```python
from build123d import *

# Parameters (mm, degrees)
F4_DEPTH = 25.4


with BuildPart() as f1:
    # F0 (on Front) → F1 (revolve)
    with BuildSketch(Plane.XZ):
        Polygon((-83.82, 18.745402), (-83.82, 14.483047), (-88.9, 14.483047), (-88.9, 34.294205), (-107.182943, 34.294205), (-177.8, -87.390703), (-177.8, -95.645703), (-162.954339, -95.645703), (-133.013525, -44.052713), (-80.645, 4.534993), (-80.645, 18.745402), align=None)
    revolve(axis=Axis((0, 0, -6.240661), (0, 0, -1)))

    # F3 (on offset) → F4 (cut)
    with BuildSketch(Plane.XY.offset(8.894205)):
        Polygon((6.35, -86.36), (6.35, -66.04), (-6.35, -66.04), (-6.35, -86.36), (-6.35, -92.71), (6.35, -92.71), align=None)
        Polygon((-54.017318, 38.519261), (-71.614954, 48.679261), (-77.114215, 51.854261), (-83.464215, 40.855739), (-77.964954, 37.680739), (-60.367318, 27.520739), align=None)
        Polygon((60.367318, 27.520739), (77.964954, 37.680739), (83.464215, 40.855739), (77.114215, 51.854261), (71.614954, 48.679261), (54.017318, 38.519261), align=None)
    extrude(amount=-F4_DEPTH, mode=Mode.SUBTRACT)


solid = f1.part
```
Design review of the part built by this model. Coordinates are the model's own, in mm. A direction names the side the tool comes from. Coordinates: 2 decimals unless noted, no trailing zeros. Loops run counter-clockwise (first coordinate to the right, second up) from the corner with the lowest first, then second, coordinate; pieces in that order, holes last. Notation, with made-up numbers: (32.25, 5) - (45.25, 5) arc R14 cw to (45.25, 31) - close; hole circle Ø2 at (1.5, -13). An arc over 180 degrees is marked (long way). Use CSV: the item, a comma, the result in double quotes. Start each with the question number.
1) Consider section D-D on z = -29. Write out the cut boundary in (x, y), then the cut area to 3 significant figures.
2) Consider section C-C on z = -73. Write out the cut boundary in (x, y), then the cut area to 3 significant figures.
3) For pin 1 Ø5 at (x, y) = (-74, 43) entering from -Z; pin 2 Ø6 at (y, z) = (-78, -57) entering from -X; pin 3 Ø3.5 at (y, z) = (-87.5, 1) entering from +X, all flat-tipped, find the tip position at first contact; note any pin that passes through.
4) Tool access review of faces 1 (the flat face through (0, -92.71, 1)), 2 (the flat face through (-40, 80, 34.294)), 3 (the flat face through (-44, 69, 18.745)): name each direction out of +Z, -Z, +X, -X, +Y, -Y from which nothing blocks a thin tool from reaching the whole face with its end or side.
5) Wall thickness on L1, parallel to Y at x = 0, z = 15 (3 decimals); L2, parallel to Z at x = 5, y = -85; L3, parallel to Y at x = 0, z = 15.5 (3 decimals): over which ranges is each line inside the solid? List them lowest first. Write a range as from..to.
6) Consider section B-B on x = 0. Write out the cut boundary in (y, z) (3 decimals).
7) The part is to be moulded in two halves that separate along X. For faces 4 (the flat face through (-78, -144, -95.646)), 5 (the conical face through (66.01, -50.62, 2.18)), 6 (the conical face through (24.19, -108.95, 26.68)), say which applies: +X half, -X half, draft (parallel to the pull), parting line (faces both ways), or undercut.
8) Consider section A-A on y = 0. Write out the cut boundary in (x, z) (3 decimals).
Geometry says:
1,outline,"circle Ø287.83 at (0, 0); hole circle Ø233.58 at (0, 0)"
1,area,"22,200 mm^2"
2,outline,"circle Ø338.9 at (0, 0); hole circle Ø299.62 at (0, 0)"
2,area,"19,700 mm^2"
3,pin 1,"z = 8.89"
3,pin 2,"x = -142.46"
3,pin 3,"x = 93.52"
4,face 1,"-Z"
4,face 2,"+Z, +X, -X, +Y, -Y"
4,face 3,"+Z"
5,L1,"-118.38..-88.9, -83.82..-80.645, 80.645..83.82, 88.9..118.38"
5,L2,"8.89..14.48"
5,L3,"-118.09..-88.9, -83.82..-80.645, 80.645..83.82, 88.9..118.09"
6,outline,"(-177.8, -95.646) - (-162.954, -95.646) - (-133.014, -44.053) - (-92.71, -6.659) - (-92.71, 8.894) - (-80.645, 8.894) - (-80.645, 18.745) - (-83.82, 18.745) - (-83.82, 14.483) - (-88.9, 14.483) - (-88.9, 34.294) - (-107.183, 34.294) - (-177.8, -87.391) - close; (80.645, 4.535) - (133.014, -44.053) - (162.954, -95.646) - (177.8, -95.646) - (177.8, -87.391) - (107.183, 34.294) - (88.9, 34.294) - (88.9, 14.483) - (83.82, 14.483) - (83.82, 18.745) - (80.645, 18.745) - close"
7,face 4,"draft"
7,face 5,"undercut"
7,face 6,"parting line"
8,outline,"(-177.8, -95.646) - (-162.954, -95.646) - (-133.014, -44.053) - (-80.645, 4.535) - (-80.645, 18.745) - (-83.82, 18.745) - (-83.82, 14.483) - (-88.9, 14.483) - (-88.9, 34.294) - (-107.183, 34.294) - (-177.8, -87.391) - close; (80.645, 4.535) - (133.014, -44.053) - (162.954, -95.646) - (177.8, -95.646) - (177.8, -87.391) - (107.183, 34.294) - (88.9, 34.294) - (88.9, 14.483) - (83.82, 14.483) - (83.82, 18.745) - (80.645, 18.745) - close"
